from build123d import *

# Parameters (mm, degrees)
ESQUISSE1_W              = 65.5
ESQUISSE1_H              = 90
BOSS_EXTRU_1_DEPTH       = 25.5
CONG_2_R                 = 2
ESQUISSE6_W              = 80
ESQUISSE6_H              = 22.5
BOSS_EXTRU_2_DEPTH       = 1.5
ENL_V_MAT_EXTRU_5_DEPTH  = 12
COQUE1_DEPTH             = 25.5
COQUE1_START             = 13
COQUE1_2_DEPTH           = 12.5
COQUE1_3_OUTLINE_W       = 3.5
COQUE1_3_OUTLINE_H       = 70
COQUE1_3_DEPTH           = 4.5
ENL_V_MAT_EXTRU_12_DEPTH = 12.5
CONG_5_R                 = 9
CONG_4_R                 = 10
BOSS_EXTRU_3_REACH       = 115.01
BOSS_EXTRU_3_END_RADIUS  = 10
ESQUISSE5_R              = 1.5
ENL_V_MAT_EXTRU_4_DEPTH  = 8
CONG_3_R                 = 6
ESQUISSE11_R             = 1.5
ENL_V_MAT_EXTRU_7_DEPTH  = 7.5
ESQUISSE12_R             = 1.5
ENL_V_MAT_EXTRU_8_DEPTH  = 7.5
ENL_V_MAT_EXTRU_9_DEPTH  = 2.5
ENL_V_MAT_EXTRU_10_DEPTH = 2.5
ENL_V_MAT_EXTRU_11_DEPTH = 2.5
BOSS_EXTRU_7_START       = -25.5
BOSS_EXTRU_7_DEPTH       = 25.5
ENL_V_MAT_EXTRU_13_DEPTH = 116.061939841
ESQUISSE21_R             = 1.5
ENL_V_MAT_EXTRU_14_DEPTH = 7.5
ENL_V_MAT_EXTRU_15_DEPTH = 2.5


# Read off the part's stored shape, not the designer's step: Coque1
with BuildPart() as part:
    # Esquisse1 → Boss.-Extru.1 (new body)
    with BuildSketch(Plane(origin=(0, 0, 0), x_dir=(1, 0, 0), z_dir=(0, 1, 0))):
        with Locations((32.75, -45)):
            Rectangle(ESQUISSE1_W, ESQUISSE1_H)
    extrude(amount=BOSS_EXTRU_1_DEPTH)

    # Congé2
    cong_2_edges = [part.edges().sort_by_distance(p)[0] for p in [
        (0, 12.75, 0),
    ]]
    fillet(cong_2_edges, radius=CONG_2_R)

    # Esquisse6 → Boss.-Extru.2 (add)
    with BuildSketch(Plane(origin=(65.5, 0, 0), x_dir=(0, 0, -1), z_dir=(1, 0, 0))):
        with Locations((-40, 11.25)):
            Rectangle(ESQUISSE6_W, ESQUISSE6_H)
    extrude(amount=BOSS_EXTRU_2_DEPTH)

    # Esquisse8 → Enlèv. mat.-Extru.5 (cut)
    with BuildSketch(Plane.XZ):
        Polygon((0, 0), (67, 0), (67, 82.382775564), (31.68341261, 28), (0, 28), align=None)
    extrude(amount=-ENL_V_MAT_EXTRU_5_DEPTH, mode=Mode.SUBTRACT)

    # Coque1 outline → Coque1 (cut)
    with BuildSketch(Plane(origin=(0, 0, 0), x_dir=(1, 0, 0), z_dir=(0, 1, 0))):
        Polygon((60.5, -90), (60.5, -81.554045593), (26.371003739, -29), (5, -29), (5, -90), align=None)
    extrude(amount=COQUE1_DEPTH, mode=Mode.SUBTRACT)

    # Coque1 2 outline → Coque1 2 (cut)
    with BuildSketch(Plane(origin=(0, 0, 0), x_dir=(1, 0, 0), z_dir=(0, 1, 0)).offset(COQUE1_START)):
        Polygon((60.5, -81.554045593), (60.5, -5), (5, -5), (5, -29), (26.371003739, -29), align=None)
    extrude(amount=COQUE1_2_DEPTH, mode=Mode.SUBTRACT)

    # Coque1 3 outline → Coque1 3 (cut)
    with BuildSketch(Plane(origin=(0, 0, 0), x_dir=(1, 0, 0), z_dir=(0, 1, 0)).offset(COQUE1_START)):
        with Locations((62.25, -40)):
            Rectangle(COQUE1_3_OUTLINE_W, COQUE1_3_OUTLINE_H)
    extrude(amount=COQUE1_3_DEPTH, mode=Mode.SUBTRACT)

    # Esquisse17 → Enlèv. mat.-Extru.12 (cut)
    with BuildSketch(Plane(origin=(0, 13, 0), x_dir=(1, 0, 0), z_dir=(0, 1, 0))):
        Polygon((5, -5), (5, -29), (26.371003739, -29), (60.5, -81.554045593), (60.5, -75), (64, -75), (64, -5), align=None)
    extrude(amount=ENL_V_MAT_EXTRU_12_DEPTH, mode=Mode.SUBTRACT)

    # Congé5
    cong_5_edges = [part.edges().sort_by_distance(p)[0] for p in [
        (64, 13, 40),
    ]]
    fillet(cong_5_edges, radius=CONG_5_R)

    # Congé4
    cong_4_edges = [part.edges().sort_by_distance(p)[0] for p in [
        (67, 12, 40),
    ]]
    fillet(cong_4_edges, radius=CONG_4_R)

    # Boss.-Extru.3: up to this cylinder (the profile starts outside it)
    boss_extru_3_end = Plane(origin=(57, 22, 72.615279), z_dir=(0, 0, -1)) * Cylinder(BOSS_EXTRU_3_END_RADIUS, 251.02, mode=Mode.PRIVATE)
    # Esquisse9 → Boss.-Extru.3 (add, up to the surface)
    with BuildSketch(Plane.XZ.offset(-12), mode=Mode.PRIVATE) as boss_extru_3_sk1:
        Polygon((57, 66.984125926), (57, 64.230008238), (66.758005852, 79.256019566), (65.5, 80.072978118), align=None)
    boss_extru_3_tool1 = extrude(boss_extru_3_sk1.sketch, amount=-BOSS_EXTRU_3_REACH, mode=Mode.PRIVATE) - boss_extru_3_end
    add(boss_extru_3_tool1.solids().sort_by_distance((61.571725, 12, 72.615279))[0])

    # Esquisse5 → Enlèv. mat.-Extru.4 (cut)
    with BuildSketch(Plane.ZY):
        with Locations((15, 17)):
            Circle(ESQUISSE5_R)
        with Locations((75, 17)):
            Circle(ESQUISSE5_R)
    extrude(amount=-ENL_V_MAT_EXTRU_4_DEPTH, mode=Mode.SUBTRACT)

    # Congé3
    cong_3_edges = [part.edges().sort_by_distance(p)[0] for p in [
        (31.68341261, 6, 28),
    ]]
    fillet(cong_3_edges, radius=CONG_3_R)

    # Esquisse11 → Enlèv. mat.-Extru.7 (cut)
    with BuildSketch(Plane(origin=(9.495472341, 0, -6.166431839), x_dir=(-0.5446390350150254, 0, -0.8386705679454252), z_dir=(0.8386705679454252, 0, -0.5446390350150254))):
        with Locations((-70.828706829, 5.5)):
            Circle(ESQUISSE11_R)
    extrude(amount=-ENL_V_MAT_EXTRU_7_DEPTH, mode=Mode.SUBTRACT)

    # Esquisse12 → Enlèv. mat.-Extru.8 (cut)
    with BuildSketch(Plane(origin=(65.5, 0, 0), x_dir=(0, 0, -1), z_dir=(1, 0, 0))):
        with Locations((-86, 20.5)):
            Circle(ESQUISSE12_R)
    extrude(amount=-ENL_V_MAT_EXTRU_8_DEPTH, mode=Mode.SUBTRACT)

    # Esquisse13 → Enlèv. mat.-Extru.9 (cut)
    with BuildSketch(Plane(origin=(5, 0, 0), x_dir=(0, 0, -1), z_dir=(1, 0, 0))):
        Polygon((-72.25, 18.58771324), (-75, 20.175426481), (-77.75, 18.58771324), (-77.75, 15.41228676), (-75, 13.824573519), (-72.25, 15.41228676), align=None)
        Polygon((-12.25, 18.58771324), (-15, 20.175426481), (-17.75, 18.58771324), (-17.75, 15.41228676), (-15, 13.824573519), (-12.25, 15.41228676), align=None)
    extrude(amount=-ENL_V_MAT_EXTRU_9_DEPTH, mode=Mode.SUBTRACT)

    # Esquisse14 → Enlèv. mat.-Extru.10 (cut)
    with BuildSketch(Plane.ZY.offset(-60.5)):
        Polygon((88.75, 22.08771324), (86, 23.675426481), (83.25, 22.08771324), (83.25, 18.91228676), (86, 17.324573519), (88.75, 18.91228676), align=None)
    extrude(amount=-ENL_V_MAT_EXTRU_10_DEPTH, mode=Mode.SUBTRACT)

    # Esquisse15 → Enlèv. mat.-Extru.11 (cut)
    with BuildSketch(Plane(origin=(5.302119501, 0, -3.443236664), x_dir=(0.5446390350150254, 0, 0.8386705679454252), z_dir=(-0.8386705679454252, 0, 0.5446390350150254))):
        Polygon((73.578706829, 3.91228676), (73.578706829, 7.08771324), (70.828706829, 8.675426481), (68.078706829, 7.08771324), (68.078706829, 3.91228676), (70.828706829, 2.324573519), align=None)
    extrude(amount=-ENL_V_MAT_EXTRU_11_DEPTH, mode=Mode.SUBTRACT)

    # Esquisse18 → Boss.-Extru.7 (add)
    with BuildSketch(Plane(origin=(0, 25.5, 0), x_dir=(1, 0, 0), z_dir=(0, 1, 0)).offset(BOSS_EXTRU_7_START)):
        Polygon((5, -90), (5, -84.920747226), (60.5, -75), (60.5, -80.079252774), align=None)
    extrude(amount=BOSS_EXTRU_7_DEPTH)

    # Esquisse19 → Enlèv. mat.-Extru.13 (cut, through all)
    with BuildSketch(Plane(origin=(0, 25.5, 0), x_dir=(1, 0, 0), z_dir=(0, 1, 0))):
        Polygon((60.5, -81.554045593), (60.5, -80.079252774), (59.641872403, -80.232644972), align=None)
    extrude(amount=-ENL_V_MAT_EXTRU_13_DEPTH, mode=Mode.SUBTRACT)

    # Esquisse21 → Enlèv. mat.-Extru.14 (cut)
    with BuildSketch(Plane(origin=(0, 0, 0), x_dir=(-1, 0, 0), z_dir=(0, 0, -1))):
        with Locations((-53, 21)):
            Circle(ESQUISSE21_R)
    extrude(amount=-ENL_V_MAT_EXTRU_14_DEPTH, mode=Mode.SUBTRACT)

    # Esquisse22 → Enlèv. mat.-Extru.15 (cut)
    with BuildSketch(Plane.XY.offset(5)):
        Polygon((53, 17.824573519), (55.75, 19.41228676), (55.75, 22.58771324), (53, 24.175426481), (50.25, 22.58771324), (50.25, 19.41228676), align=None)
    extrude(amount=-ENL_V_MAT_EXTRU_15_DEPTH, mode=Mode.SUBTRACT)


solid = part.part
Geometry check sheet. Reference: the model listing, model coordinates, mm. A direction names the side the tool comes from. Round coordinates to 2 decimals unless told otherwise and drop trailing zeros. Loops run counter-clockwise (first coordinate to the right, second up) from the corner with the lowest first, then second, coordinate; pieces in that order, holes last. Notation, with made-up numbers: (89, -27.75) - (97, -27.75) arc R7 cw to (97, -18.75) - close; hole circle Ø1 at (71, 66). An arc over 180 degrees is marked (long way). One line per question, with ' | ' between items. Start each with the question number.
1. Cross-section at B-B on x = 23. Record the cut outline in (y, z), then the cut area to 3 significant figures.
2. Scan lines: line 1 (Y direction, x = 53, z = 1); line 2 (Y direction, x = 1, z = 75); line 3 (Y direction, x = 18, z = 19.5). Record each from-to range of solid material in increasing order. Write a range as [from, to].
3. Tool access check on faces 4 (the face through (51.606, 18.63, 3.768)), 5 (the face through (35, 13, 23)), 6 (the face through (0, 13, 56)), 7 (the face through (16, 6, 29)). Record the directions out of +Z, -Z, +X, -X, +Y, -Y that give a thin tool (end or side, any length) a straight path to the whole face; none if there is none.
4. Depth check by flat-ended pin: pin 1 (1.6 mm diameter, centred on x = 54.5, y = 20, fed in from +Z); pin 2 (1 mm diameter, centred on x = 19.5, y = 6.5, fed in from +Z); pin 3 (0.8 mm diameter, centred on y = 21.5, z = 3.5, fed in from +X); pin 4 (8 mm diameter, centred on x = 14, z = 11.5, fed in from +Y). Enter the tip coordinate at first touch or a pass-through.
5. Cross-section at A-A on z = 27. Record the cut outline in (x, y).
6. Draft check along Z on faces 1 (the face through (49.703, 5.916, 55.748)), 2 (the face through (63, 19, 85)), 3 (the face through (63, 13, 90)). Enter one of: released by +Z, released by -Z, zero draft, split by the parting line, or undercut.
7. Cross-section at C-C on z = 37.5. Record the cut outline in (x, y).
Taken from the geometry:
1) outline: (0, 28) - (12, 28) - (12, 0) - (25.5, 0) - (25.5, 5) - (13, 5) - (13, 29) - (0, 29) - close; (0, 81.7) - (25.5, 81.7) - (25.5, 86.78) - (0, 86.78) - close | area: 233 mm²
2) line 1: [12, 19.5], [22.5, 25.5] | line 2: [0, 15.5], [18.5, 25.5] | line 3: [12, 13]
3) face 4: none | face 5: +Y | face 6: +Z, -Z, -X, +Y, -Y | face 7: +Y, -Y
4) pin 1: z = 81.29 | pin 2: z = 87.5 | pin 3: x = 67 | pin 4: y = 13
5) outline: (0, 12) - (57, 12) arc R10 ccw to (67, 22) - (67, 22.5) - (65.5, 22.5) - (65.5, 25.5) - (64, 25.5) - (64, 22) arc R9 cw to (55, 13) - (5, 13) - (5, 25.5) - (0, 25.5) - close
6) face 1: released by -Z | face 2: undercut | face 3: released by +Z
7) outline: (0, 0) - (5, 0) - (5, 25.5) - (0, 25.5) - close; (31.89, 0) - (37.85, 0) - (37.85, 12) - (57, 12) arc R10 ccw to (67, 22) - (67, 22.5) - (65.5, 22.5) - (65.5, 25.5) - (64, 25.5) - (64, 22) arc R9 cw to (55, 13) - (31.89, 13) - close
